Check sheet for the modelled part. Datum: model origin and axes. Units: mm. Face numbers are marked on the shaded views. A direction names the side the tool comes from. Give positions to 0.01 mm unless a question says otherwise; leave off trailing zeros. Loops run counter-clockwise (first coordinate to the right, second up) from the corner with the lowest first, then second, coordinate; pieces in that order, holes last. Notation, with made-up numbers: (43.5, 11) -> (74.5, 11) arc R21 ccw to (74.5, 35) -> close; hole circle Ø1 at (-34.75, -8). An arc over 180 degrees is marked (long way). Write each question's results on one line, items separated by ' | '. Start each with the question number.
Item 1: Scan lines: line 1 along Z through (x, y) = (-3.75, -4.25); line 2 along X through (y, z) = (2, 23); line 3 along Z through (x, y) = (-4.75, 5.5). Record each from-to range of solid material in increasing order.
Item 2: Cross-section at C-C on z = 26. Enter the section's corners in (x, y), then the cut area to 3 significant figures.
Item 3: Cross-section at D-D on z = 5. Enter the section's corners in (x, y), then the cut area to 3 significant figures.
Item 4: Cross-section at A-A on y = 0. Enter the section's corners in (x, z).
Item 5: Gauge pin test, flat ends, axial feed: pin 1 Ø1 at (y, z) = (-0.5, 31) entering from +X; pin 2 Ø1 at (y, z) = (-2.5, 9.5) entering from +X; pin 3 Ø4 at (x, z) = (-5, 14.5) entering from -Y. Record the tip position at first contact, or that the pin passes through.
Item 6: Access from +Z, -Z, +X, -X, +Y, -Y to the whole of each face (thin tool, end or side, straight path). Record for the marked faces 1 and 2.
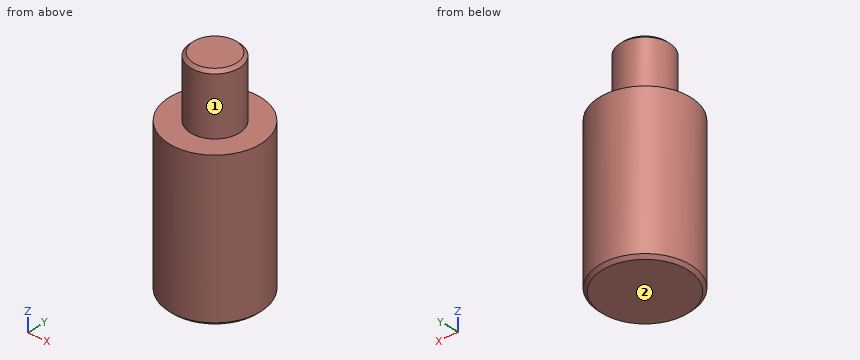
Autodesk Inventor part; units mm, degrees
ref_plane "YZ Plane" through (0, 0, 0) normal (1, 0, 0) x (0, 1, 0)
ref_plane "XZ Plane" through (0, 0, 0) normal (0, 1, 0) x (-1, 0, 0)
ref_plane "XY Plane" through (0, 0, 0) normal (0, 0, 1) x (1, 0, 0)
sketch "Schizzo1" plane through (0, 0, 0) normal (0, 0, 1) x (1, 0, 0)
  circle A0 centre (0, 0) radius 7.5
  dimension "d0" = 15
extrude "Estrusione1" add sketch "Schizzo1" along normal blind 25
sketch "Schizzo2" plane through (0, 0, 25) normal (0, 0, 1) x (1, 0, 0)
  circle A0 centre (0, 0) radius 4
  dimension "d3" = 8
extrude "Estrusione2" add sketch "Schizzo2" along normal blind 10
chamfer "Smusso1" distance 0.5 angle 45 2 edges at (-4, 0, 35) (-7.5, 0, 0)
thread "Filettatura2"
properties part number "Perno tendi motore" material "Acciaio inossidabile"
Answer sheet:
1) line 1: z = 0 to 25 | line 2: x = -7.23 to 7.23 | line 3: z = 0.27 to 25
2) outline: circle Ø8 at (0, 0) | area: 50.3 mm²
3) outline: circle Ø15 at (0, 0) | area: 177 mm²
4) outline: (-7.5, 0.5) -> (-7, 0) -> (7, 0) -> (7.5, 0.5) -> (7.5, 25) -> (4, 25) -> (4, 34.5) -> (3.5, 35) -> (-3.5, 35) -> (-4, 34.5) -> (-4, 25) -> (-7.5, 25) -> close
5) pin 1: stops at x = 4 | pin 2: stops at x = 7.23 | pin 3: stops at y = -6.87
6) face 1: +Z | face 2: -Z, +X, -X, +Y, -Y
